Geometry: final body of the model. Coordinates: model frame, mm. Round coordinates to 2 decimals unless told otherwise and drop trailing zeros. Loops run counter-clockwise (first coordinate to the right, second up) from the corner with the lowest first, then second, coordinate; pieces in that order, holes last. Notation, with made-up numbers: M 59.25,45 L 91.25,45 A8 ccw 91.25,50 Z; hole C 69.5,72.5 d5. An arc over 180 degrees is marked long. Return JSON: item names as keys, results as strings.
Autodesk Inventor part; units mm, degrees
ref_plane "Work Plane1" through (0, 300, 0) normal (0, 1, 0) x (1, 0, 0)
ref_plane "YZ Plane" through (0, 0, 0) normal (1, 0, 0) x (0, 1, 0)
ref_plane "XZ Plane" through (0, 0, 0) normal (0, 1, 0) x (-1, 0, 0)
sketch "Sketch1" plane through (0, 0, 0) normal (0, 1, 0) x (-1, 0, 0)
  line L0 (-5, -5) -> (5, -5)
  line L1 (5, -5) -> (5, 5)
  line L2 (5, 5) -> (-5, 5)
  line L3 (-5, 5) -> (-5, -5)
  line L4 (-5, -5) -> (5, 5) construction
  line L5 (5, -5) -> (-5, 5) construction
  line L6 (-4, -4) -> (4, -4)
  line L7 (4, -4) -> (4, 4)
  line L8 (4, 4) -> (-4, 4)
  line L9 (-4, 4) -> (-4, -4)
  line L10 (-4, -4) -> (4, 4) construction
  line L11 (4, -4) -> (-4, 4) construction
  point P0 (0, 0)
  dimension "d0" = 10
  dimension "d1" = 10
  dimension "d2" = 8
  dimension "d3" = 8
extrude "Extrusion1" add sketch "Sketch1" along normal blind 600
sketch "Sketch2" plane through (5, 0, -5) normal (1, 0, 0) x (0, 0, -1)
  line L0 (-10, 600) -> (0, 600)
  point P0 (-5, 0)
  point P1 (-5, 545)
  point P2 (-5, 525)
  point P3 (-5, 590)
  point P4 (-5, 555)
  point P5 (-5, 575)
  dimension "d6" = 55
  dimension "d7" = 20
  dimension "d21" = 10
  dimension "d23" = 35
  dimension "d24" = 15
hole "Hole1" at (5, 545, 0) at (5, 525, 0) at (5, 590, 0) at (5, 555, 0) at (5, 575, 0) direction (-1, 0, 0) diameter 3 depth 80.45
sketch "Sketch3" plane through (-5, 0, -5) normal (0, 0, -1) x (-1, 0, 0)
  line L0 (-10, 600) -> (0, 600)
  circle A0 centre (-5, 595) radius 1.5
  line L1 (-10, 0) -> (0, 0)
  circle A1 centre (-5, 5) radius 1.75
  circle A2 centre (-5, 60) radius 1.75
  point P0 (-5, 0)
  dimension "d15" = 5
  dimension "d16" = 3
  dimension "d19" = 5
  dimension "d20" = 3.5
  dimension "d25" = 55
extrude "Extrusion2" cut sketch "Sketch3" against normal blind 600
ref_plane "Work Plane1" through (0, 300, 0) normal (0, 1, 0) x (1, 0, 0)
mirror "Mirror1" about plane through (0, 300, 0) normal (0, 1, 0) of "Hole1"
properties part number "10x10x600" material "アルミニウム 6061"
Q1. Section query A-A (x = 0). State how many separate pieces and enclosed holes the cut face has, plus the area to 3 significant figures.
Determined:
{"separate pieces": "8", "enclosed holes": "0", "area": "1,180 mm^2"}
Q2. Material intervals for L1, parallel to Y at x = 0, z = -4.2; L2, parallel to Z at x = -4.55, y = 10; L3, parallel to X at y = 330, z = 3, sorted ascending.
Determined:
{"L1": "y = 0 to 3.25, 6.75 to 58.25, 61.75 to 593.5, 596.5 to 600", "L2": "z = -5 to -1.5, 1.5 to 5", "L3": "x = -5 to -4, 4 to 5"}
Q3. Pin query (flat end, axial travel): pin 1 (1.8 mm diameter, centred on y = 575, z = 0, fed in from +X); pin 2 (3.5 mm diameter, centred on y = 10, z = 0, fed in from +X). Return the tip coordinate at first contact, or that it passes through.
Determined:
{"pin 1": "passes through", "pin 2": "stops at x = 5"}
Q4. Section query B-B (y = 82). Output: boundary loops of the cut face in (x, z).
Determined:
{"outline": "M -5,-5 L 5,-5 L 5,5 L -5,5 Z; hole M -4,-4 L 4,-4 L 4,4 L -4,4 Z"}
